```python
from build123d import *

# Parameters (mm, degrees)
F0_W     = 220
F0_H     = 275.358058
F0_R     = 2.5
F1_DEPTH = 10
F2_DEPTH = 10
F3_R     = 3
F4_DEPTH = 20


with BuildPart() as f1:
    # F0 (on Front) → F1 (new body)
    with BuildSketch(Plane.XZ):
        with Locations((0, -5.406313)):
            Rectangle(F0_W, F0_H)
        with Locations((-90.25, 7.272716)):
            Circle(F0_R, mode=Mode.SUBTRACT)
        with Locations((-59.75, 7.272716)):
            Circle(F0_R, mode=Mode.SUBTRACT)
        with Locations((-90.25, 107.272716)):
            Circle(F0_R, mode=Mode.SUBTRACT)
        with Locations((-59.75, 107.272716)):
            Circle(F0_R, mode=Mode.SUBTRACT)
        with Locations((59.75, 7.272716)):
            Circle(F0_R, mode=Mode.SUBTRACT)
        with Locations((90.25, 7.272716)):
            Circle(F0_R, mode=Mode.SUBTRACT)
        with Locations((59.75, 107.272716)):
            Circle(F0_R, mode=Mode.SUBTRACT)
        with Locations((90.25, 107.272716)):
            Circle(F0_R, mode=Mode.SUBTRACT)
        with Locations((-90.25, 107.272716)):
            Circle(F0_R)
        with Locations((-59.75, 107.272716)):
            Circle(F0_R)
        with Locations((-90.25, 7.272716)):
            Circle(F0_R)
        with Locations((-59.75, 7.272716)):
            Circle(F0_R)
        with Locations((59.75, 7.272716)):
            Circle(F0_R)
        with Locations((90.25, 7.272716)):
            Circle(F0_R)
        with Locations((59.75, 107.272716)):
            Circle(F0_R)
        with Locations((90.25, 107.272716)):
            Circle(F0_R)
    extrude(amount=-F1_DEPTH)

    # F0 (on Front) → F2 (join)
    with BuildSketch(Plane.XZ):
        with Locations((90.25, 107.272716)):
            Circle(F0_R)
        with Locations((59.75, 107.272716)):
            Circle(F0_R)
        with Locations((-59.75, 107.272716)):
            Circle(F0_R)
        with Locations((-90.25, 107.272716)):
            Circle(F0_R)
        with Locations((90.25, 7.272716)):
            Circle(F0_R)
        with Locations((59.75, 7.272716)):
            Circle(F0_R)
        with Locations((-90.25, 7.272716)):
            Circle(F0_R)
        with Locations((-59.75, 7.272716)):
            Circle(F0_R)
    extrude(amount=F2_DEPTH)

    # F3 (on face) → F4 (join)
    with BuildSketch(Plane.XZ):
        with Locations((35, -103.085342)):
            Circle(F3_R)
        with Locations((35, -123.085342)):
            Circle(F3_R)
        with Locations((-35, -123.085342)):
            Circle(F3_R)
        with Locations((-35, -103.085342)):
            Circle(F3_R)
    extrude(amount=-F4_DEPTH)


solid = f1.part
```
Check sheet for the modelled part. Datum: model origin and axes. Units: mm. A direction names the side the tool comes from. Give positions to 0.01 mm unless a question says otherwise; leave off trailing zeros. Loops run counter-clockwise (first coordinate to the right, second up) from the corner with the lowest first, then second, coordinate; pieces in that order, holes last. Notation, with made-up numbers: M -34.75,-14 L 15.25,-14 A33 ccw 15.25,15 Z; hole C 76.5,-39 d4. An arc over 180 degrees is marked long. Answer as CSV lines item,"result".
Item 1: Scan lines: L1, parallel to X at y = -5.5, z = 9; L2, parallel to Y at x = -24.5, z = -110; L3, parallel to Z at x = -36, y = 12.5. Record each from-to range of solid material in increasing order.
Reply:
L1,"-92.06 to -88.44, -61.56 to -57.94, 57.94 to 61.56, 88.44 to 92.06"
L2,"0 to 10"
L3,"-125.91 to -120.26, -105.91 to -100.26"
Item 2: Sectioned sample at A-A, the plane y = -6.25. Enter the section's corners in (x, z), then the cut area to 3 significant figures.
Reply:
outline,"C -90.25,7.27 d5; C -90.25,107.27 d5; C -59.75,7.27 d5; C -59.75,107.27 d5; C 59.75,7.27 d5; C 59.75,107.27 d5; C 90.25,7.27 d5; C 90.25,107.27 d5"
area,"157 mm^2"
Item 3: Sectioned sample at B-B, the plane x = 35. Enter the section's corners in (y, z), then the cut area to 3 significant figures.
Reply:
outline,"M 0,-143.09 L 10,-143.09 L 10,-126.09 L 20,-126.09 L 20,-120.09 L 10,-120.09 L 10,-106.09 L 20,-106.09 L 20,-100.09 L 10,-100.09 L 10,132.27 L 0,132.27 Z"
area,"2,870 mm^2"
Item 4: Depth check by flat-ended pin: pin 1 Ø1.5 at (y, z) = (-1.5, 43) entering from +X; pin 2 Ø6 at (x, z) = (-39, -89.5) entering from +Y; pin 3 Ø8 at (x, z) = (-75, -98) entering from -Y. Enter the tip coordinate at first touch or a pass-through.
Reply:
pin 1,"through"
pin 2,"y = 10"
pin 3,"y = 0"
Item 5: Draft check along Z on faces 3 (the face through (110, 5, -7)), 4 (the face through (-2, 5, 132.273)), 5 (the face through (32.789, 14.93, -121.058)), 6 (the face through (32, 15, -103)). Enter one of: pulls with the +Z half, pulls with the -Z half, needs draft (parallel to the pull), parting line crosses it, or undercut.
Reply:
face 3,"needs draft"
face 4,"pulls with the +Z half"
face 5,"undercut"
face 6,"undercut"
Item 6: Sectioned sample at D-D, the plane y = 16.25. Enter the section's corners in (x, z), then the cut area to 3 significant figures.
Reply:
outline,"C -35,-123.09 d6; C -35,-103.09 d6; C 35,-123.09 d6; C 35,-103.09 d6"
area,"113 mm^2"
Item 7: Sectioned sample at C-C, the plane z = -43. Enter the section's corners in (x, y).
Reply:
outline,"M -110,0 L 110,0 L 110,10 L -110,10 Z"
Item 8: Set-up check for faces 1 (the face through (-38, 15, -103)), 2 (the face through (-2, 5, -143.085)): record each of +Z, -Z, +X, -X, +Y, -Y from which the full face is reachable in a straight line by a thin tool's end or side.
Reply:
face 1,"+Y"
face 2,"-Z, +X, -X, +Y, -Y"
